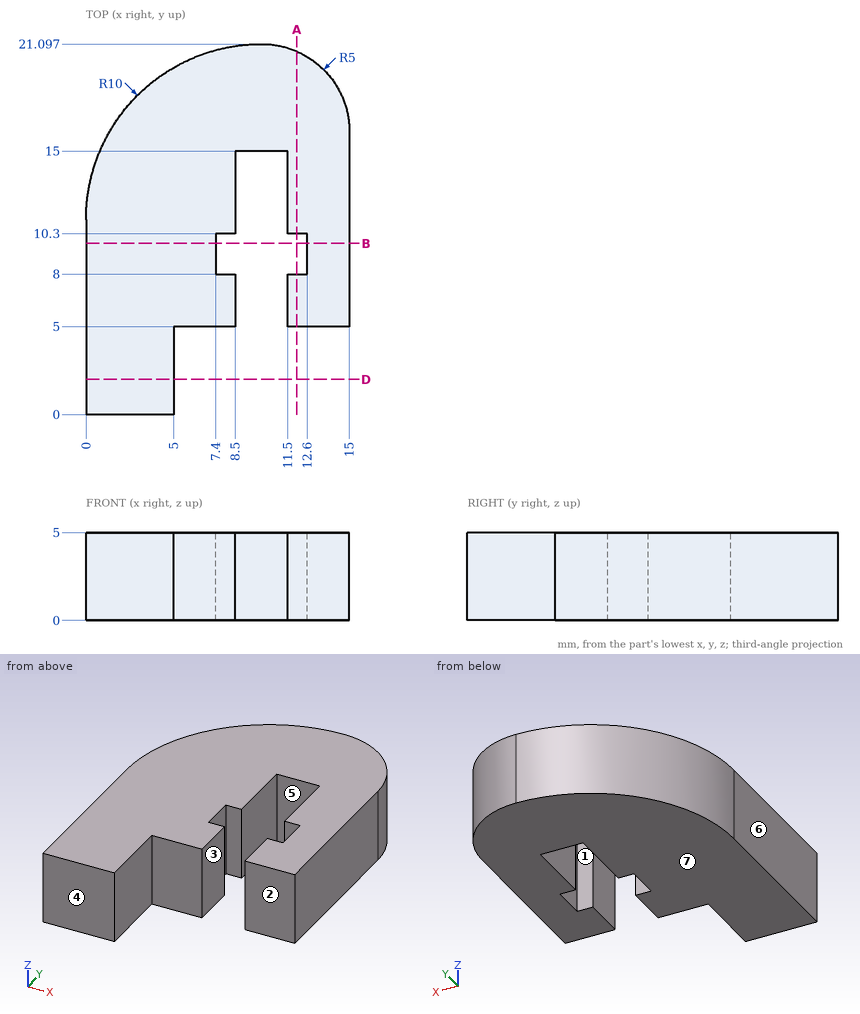
Job drawing, mm, ordinate dimensions from the low corner. One solid piece. A direction names the side the tool comes from. Give positions to 0.01 mm unless a question says otherwise; leave off trailing zeros. Write each loop counter-clockwise with the first axis right and the second up, starting at its lowest first coordinate (ties: lowest second). Pieces come first, ordered by that corner, then holes. Notation, with made-up numbers: (-33, -12) - (-15, -12) arc R18 ccw to (-15, 7) - close; hole circle Ø2 at (-6.5, -22). An arc over 180 degrees is marked (long way). Use one line per item in the form item = value. Start each with the question number.
1. Band-saw the part on A-A on x = 12. Write the cut outline in (y, z), plus the area to 3 significant figures.
2. Drop flat-ended pins along their axis: pin 1 Ø1.5 at (y, z) = (16.5, 4.5) entering from -X; pin 2 Ø1.2 at (x, z) = (12.5, 2) entering from -Y. Give the stop position or say it passes through.
3. Probe line 1 (X direction, y = 7.5, z = 0.85); line 2 (X direction, y = 10, z = 1); line 3 (Y direction, x = 9.75, z = 2.7) (1 decimal). List the from-to ranges inside material, lowest first. Write a range as [from, to].
4. Band-saw the part on D-D on y = 2. Write the cut outline in (x, z).
5. Two-plate mould, pull along X, no slides. Class the marked faces 5, 6 and 7: released by +X, released by -X, zero draft, split by the parting line, or undercut.
6. Band-saw the part on B-B on y = 9.75. Write the cut outline in (x, z), plus the area to 3 significant figures.
7. 3-axis set-ups, long thin cutter, end or side, ignore diameter. For the marked faces 1, 2, 3 and 4: which of +Z, -Z, +X, -X, +Y, -Y reach the whole face in a straight line?
Conclusion:
q1.outline = (5, 0) - (8, 0) - (8, 5) - (5, 5) - close; (10.3, 0) - (20.68, 0) - (20.68, 5) - (10.3, 5) - close
q1.area = 66.9 mm²
q2.pin_1 = 1.15
q2.pin_2 = 5
q3.line_1 = [0, 8.5], [11.5, 15]
q3.line_2 = [0, 7.4], [12.6, 15]
q3.line_3 = [15, 21.1]
q4.outline = (0, 0) - (5, 0) - (5, 5) - (0, 5) - close
q5.face_5 = undercut
q5.face_6 = released by -X
q5.face_7 = zero draft
q6.outline = (0, 0) - (7.4, 0) - (7.4, 5) - (0, 5) - close; (12.6, 0) - (15, 0) - (15, 5) - (12.6, 5) - close
q6.area = 49.0 mm²
q7.face_1 = +Z, -Z
q7.face_2 = +Z, -Z, +X, -Y
q7.face_3 = +Z, -Z, -Y
q7.face_4 = +Z, -Z, +X, -X, -Y
